Input: part model. Units: mm. Frame: model coordinates. A direction names the side the tool comes from. Give positions to 0.01 mm unless a question says otherwise; leave off trailing zeros. Loops run counter-clockwise (first coordinate to the right, second up) from the corner with the lowest first, then second, coordinate; pieces in that order, holes last. Notation, with made-up numbers: (18, -6.5) - (54, -6.5) arc R10 cw to (54, 3.5) - close; hole circle Ø4 at (-22.5, -2.5). An arc over 180 degrees is marked (long way). Answer as a JSON object with one key per item and string values.
from build123d import *

# Parameters (mm, degrees)
SKICA1_W                 = 30
SKICA1_H                 = 67
SKICA1_R                 = 1
P_IDAT_VYSUNUT_M1_DEPTH  = 1.3
ODEBRAT_VYSUNUT_M1_DEPTH = 1.3
ZKOSEN_1_SIZE            = 2
SCALA1_SCALE             = 0.64


with BuildPart() as part:
    # Skica1 → Přidat vysunutím1 (new body)
    with BuildSketch(Plane.XY):
        with Locations((0, -3.5)):
            Rectangle(SKICA1_W, SKICA1_H)
        with Locations((-11.5, 15)):
            Circle(SKICA1_R, mode=Mode.SUBTRACT)
        with Locations((-11.5, -15)):
            Circle(SKICA1_R, mode=Mode.SUBTRACT)
        with Locations((11.5, -15)):
            Circle(SKICA1_R, mode=Mode.SUBTRACT)
        with Locations((11.5, 15)):
            Circle(SKICA1_R, mode=Mode.SUBTRACT)
    extrude(amount=P_IDAT_VYSUNUT_M1_DEPTH)

    # Skica2 → Odebrat vysunutím1 (cut)
    with BuildSketch(Plane.XY.offset(1.3)):
        Polygon((-15, 12.5), (-15, 17.5), (-15, 30), (-13, 30), (-7, 30), (0, 30), (0, 36.174813822), (-21.495608396, 36.174813822), (-21.495608396, -40.537143206), (0, -40.537143206), (0, -37), (-7, -37), (-13, -37), (-15, -37), (-15, -17.5), (-15, -12.5), align=None)
        Polygon((0, 36.174813822), (0, 30), (7, 30), (13, 30), (15, 30), (15, 17.5), (15, 12.5), (15, -12.5), (15, -17.5), (15, -37), (13, -37), (7, -37), (0, -37), (0, -40.537143206), (21.495608396, -40.537143206), (21.495608396, 36.174813822), align=None)
        Polygon((15, 30), (13, 30), (13, 19.5), (15, 17.5), align=None)
        Polygon((15, -12.5), (15, 12.5), (13, 10.5), (13, -10.5), align=None)
        Polygon((13, -19.5), (13, -37), (15, -37), (15, -17.5), align=None)
        Polygon((0, -35), (0, -37), (7, -37), (5, -35), align=None)
        Polygon((-5, -35), (-7, -37), (0, -37), (0, -35), align=None)
        Polygon((-13, -19.5), (-15, -17.5), (-15, -37), (-13, -37), align=None)
        Polygon((-13, 10.5), (-15, 12.5), (-15, -12.5), (-13, -10.5), align=None)
        Polygon((-15, 30), (-15, 17.5), (-13, 19.5), (-13, 30), align=None)
        Polygon((7, 30), (0, 30), (0, 28), (5, 28), align=None)
        Polygon((0, 30), (-7, 30), (-5, 28), (0, 28), align=None)
        with BuildLine():
            Line((-7.5, 23), (-7.5, 5))
            ThreePointArc((-7.5, 5), (-5, 2.5), (-2.5, 5))
            Line((-2.5, 5), (-2.5, 23))
            ThreePointArc((-2.5, 23), (-5, 25.5), (-7.5, 23))
        make_face()
        with BuildLine():
            ThreePointArc((7.5, 5), (5, 2.5), (2.5, 5))
            Line((2.5, 5), (2.5, 23))
            ThreePointArc((2.5, 23), (5, 25.5), (7.5, 23))
            Line((7.5, 23), (7.5, 5))
        make_face()
        with BuildLine():
            ThreePointArc((7.5, -30), (5, -32.5), (2.5, -30))
            Line((2.5, -30), (2.5, -5))
            ThreePointArc((2.5, -5), (5, -2.5), (7.5, -5))
            Line((7.5, -5), (7.5, -30))
        make_face()
        with BuildLine():
            Line((-7.5, -5), (-7.5, -30))
            ThreePointArc((-7.5, -30), (-5, -32.5), (-2.5, -30))
            Line((-2.5, -30), (-2.5, -5))
            ThreePointArc((-2.5, -5), (-5, -2.5), (-7.5, -5))
        make_face()
    extrude(amount=-ODEBRAT_VYSUNUT_M1_DEPTH, mode=Mode.SUBTRACT)

    # Zkosení1
    zkosen_1_edges = [part.edges().sort_by_distance(p)[0] for p in [
        (13, 30, 0.65),
        (-13, 30, 0.65),
        (-13, -37, 0.65),
        (13, -37, 0.65),
    ]]
    chamfer(zkosen_1_edges, length=ZKOSEN_1_SIZE)


with BuildPart() as part_1:
    # Scala1: scaled about (0, -3.201388425, 0.65)
    add(part.part.scale(SCALA1_SCALE).moved(Location((0, -1.152499833, 0.234))))


solid = part_1.part
Item 1: Cut plane D-D (z = 0.7). Give the number of separate pieces and of enclosed holes in the cut face, then the cut area to 3 significant figures.
Geometry check:
{"separate pieces": "1", "enclosed holes": "8", "area": "500 mm2"}
Item 2: Cut plane B-B (x = 4). Return loops of the section in (y, z).
Geometry check:
{"outline": "(-24.35, 0.23) - (-21.74, 0.23) - (-21.74, 1.07) - (-24.35, 1.07) - close; (-2.97, 0.23) - (0.66, 0.23) - (0.66, 1.07) - (-2.97, 1.07) - close; (14.95, 0.23) - (17.57, 0.23) - (17.57, 1.07) - (14.95, 1.07) - close"}
Item 3: Access query for faces 1 (the face through (8.95, -8.5, 0.66)), 2 (the face through (-8.95, 6.2, 0.66)), 3 (the face through (3.24, 0.45, 0.66)). Directions: +Z, -Z, +X, -X, +Y, -Y. A direction counts if a zero-diameter tool reaches every point of the face in a straight line with its end or side. Return the directions, or none.
Geometry check:
{"face 1": "+Z, -Z, +X", "face 2": "+Z, -Z, -X", "face 3": "+Z, -Z"}
Item 4: Cut plane A-A (y = 13). Return loops of the section in (x, z), then the cut area to 3 significant figures.
Geometry check:
{"outline": "(-8.32, 0.23) - (-4.8, 0.23) - (-4.8, 1.07) - (-8.32, 1.07) - close; (-1.6, 0.23) - (1.6, 0.23) - (1.6, 1.07) - (-1.6, 1.07) - close; (4.8, 0.23) - (8.32, 0.23) - (8.32, 1.07) - (4.8, 1.07) - close", "area": "8.52 mm2"}
Item 5: Cut plane C-C (y = -2). Return loops of the section in (x, z), then the cut area to 3 significant figures.
Geometry check:
{"outline": "(-8.32, 0.23) - (8.32, 0.23) - (8.32, 1.07) - (-8.32, 1.07) - close", "area": "13.8 mm2"}
Item 6: Material intervals for line 1 (X direction, y = -16.5, z = 0.95); line 2 (X direction, y = 10, z = 0.5); line 3 (Y direction, x = -4.25, z = 0.3), sorted ascending. Write a range as [from, to].
Geometry check:
{"line 1": "x = [-8.32, -4.8], [-1.6, 1.6], [4.8, 8.32]", "line 2": "x = [-9.6, -4.8], [-1.6, 1.6], [4.8, 9.6]", "line 3": "y = [-24.6, -21.56], [-3.15, 0.84], [14.77, 17.82]"}
Item 7: Mould query, pull axis Y, two halves, no side actions, for faces 4 (the face through (-3.85, 17.42, 0.66)), 5 (the face through (3.165, -2.753, 0.656)), 6 (the face through (8.32, 14.1, 0.7)), 7 (the face through (8.32, -1.1, 0.7)). Classes: released by +Y, released by -Y, zero draft, split by the parting line, or undercut.
Geometry check:
{"face 4": "released by +Y", "face 5": "undercut", "face 6": "zero draft", "face 7": "undercut"}
